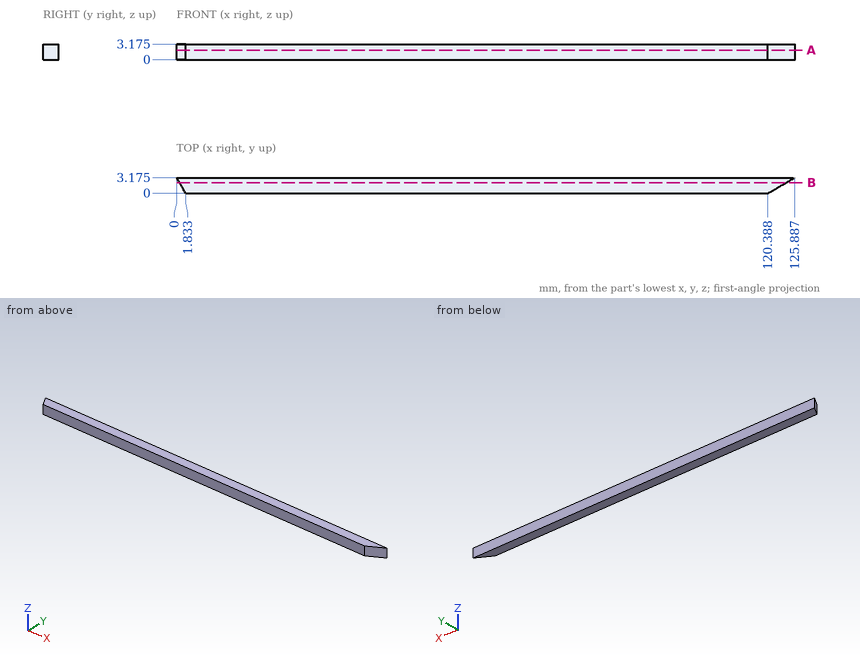
The figure shows three views and two pictorial views of one solid part (mm, origin at its lowest corner). Answer the questions. Coordinates: 2 decimals unless noted, no trailing zeros. Order: outer loops, then holes, each group sorted by start corner. A loop starts at its lowest first (then second) coordinate and runs counter-clockwise, first axis right, second up. Notation, with made-up numbers: M 48.5,-27.75 L 76.5,-27.75 A29 cw 76.5,4.25 Z; hole C -24.5,34.25 d4. An arc over 180 degrees is marked long. Use CSV: the item, a comma, the result in double quotes.
1) A flat-ended cylindrical pin translates along its axis: pin 1 Ø1 at (y, z) = (2.5, 2) entering from -X. Find the tip coordinate at first contact, or state that the pin passes through.
Worked out:
pin 1,"stops at x = 0.1"
2) Section B-B on y = 2.15 is taken. Write down the section's boundary in (x, z) (1 decimal), plus the area to 3 significant figures.
Worked out:
outline,"M 0.6,0 L 124.1,0 L 124.1,3.2 L 0.6,3.2 Z"
area,"392 mm^2"
3) Section A-A on z = 1.95 is taken. Write down the section's boundary in (x, y) (1 decimal), plus the area to 3 significant figures.
Worked out:
outline,"M 0,3.2 L 1.8,0 L 120.4,0 L 125.9,3.2 Z"
area,"388 mm^2"
4) Consider line 1 (X direction, y = 2.6, z = 1.2); line 2 (X direction, y = 3.05, z = 2.25). Determine where each line is inside the solid, lowest interval first. Write a range as [from, to].
Worked out:
line 1,"x = [0.33, 124.89]"
line 2,"x = [0.07, 125.67]"
